```python
from build123d import *

# Parameters (mm, degrees)
F0_R      = 8.37282
F0_R_2    = 8.3693
F1_DEPTH  = 19.05
F2_W      = 20.754474
F2_H      = 61.66184
F3_DEPTH  = 25.4
F5_DEPTH  = 25.4
F7_DEPTH  = 12.7
F6_R      = 3.8309
F8_DEPTH  = 15.24
F10_DEPTH = 12.7
F9_R      = 3.8354
F11_DEPTH = 15.24


with BuildPart() as f1:
    # F0 (on Top) → F1 (new body)
    with BuildSketch(Plane.XY):
        with BuildLine():
            Line((-15.24, 50.8), (-15.24, 0))
            Line((-15.24, 0), (-15.24, -50.8))
            ThreePointArc((-15.24, -50.8), (0, -66.04), (15.24, -50.8))
            Line((15.24, -50.8), (15.24, 0))
            Line((15.24, 0), (15.24, 50.8))
            ThreePointArc((15.24, 50.8), (0, 66.04), (-15.24, 50.8))
        make_face()
        with Locations((0, -50.8)):
            Circle(F0_R, mode=Mode.SUBTRACT)
        with Locations((0, 50.8)):
            Circle(F0_R_2, mode=Mode.SUBTRACT)
    extrude(amount=F1_DEPTH)

    # F2 (on face) → F3 (join)
    with BuildSketch(Plane.XY.offset(19.05)):
        Rectangle(F2_W, F2_H)
    extrude(amount=F3_DEPTH)

    # F4 (on face) → F5 (cut)
    with BuildSketch(Plane.YZ.offset(10.377237)):
        with BuildLine():
            Line((18.13092, 44.45), (-18.13092, 44.45))
            ThreePointArc((-18.13092, 44.45), (0, 27.163165), (18.13092, 44.45))
        make_face()
    extrude(amount=-F5_DEPTH, mode=Mode.SUBTRACT)

    # F6 (on face) → F7 (join)
    with BuildSketch(Plane.XZ.offset(30.83092)):
        with BuildLine():
            Line((3.8309, 44.45), (10.377237, 44.45))
            ThreePointArc((10.377237, 44.45), (0, 54.827237), (-10.377237, 44.45))
            Line((-10.377237, 44.45), (-3.8309, 44.45))
            ThreePointArc((-3.8309, 44.45), (0, 48.2809), (3.8309, 44.45))
        make_face()
    extrude(amount=-F7_DEPTH)

    # F6 (on face) → F8 (cut)
    with BuildSketch(Plane.XZ.offset(30.83092)):
        with Locations((0, 44.45)):
            Circle(F6_R)
    extrude(amount=-F8_DEPTH, mode=Mode.SUBTRACT)

    # F9 (on face) → F10 (join)
    with BuildSketch(Plane(origin=(0, 30.83092, 0), x_dir=(-1, 0, 0), z_dir=(0, 1, 0))):
        with BuildLine():
            Line((3.8354, 44.45), (10.377237, 44.45))
            ThreePointArc((10.377237, 44.45), (0, 54.827237), (-10.377237, 44.45))
            Line((-10.377237, 44.45), (-3.8354, 44.45))
            ThreePointArc((-3.8354, 44.45), (0, 48.2854), (3.8354, 44.45))
        make_face()
    extrude(amount=-F10_DEPTH)

    # F9 (on face) → F11 (cut)
    with BuildSketch(Plane(origin=(0, 30.83092, 0), x_dir=(-1, 0, 0), z_dir=(0, 1, 0))):
        with Locations((0, 44.45)):
            Circle(F9_R)
    extrude(amount=-F11_DEPTH, mode=Mode.SUBTRACT)


solid = f1.part
```
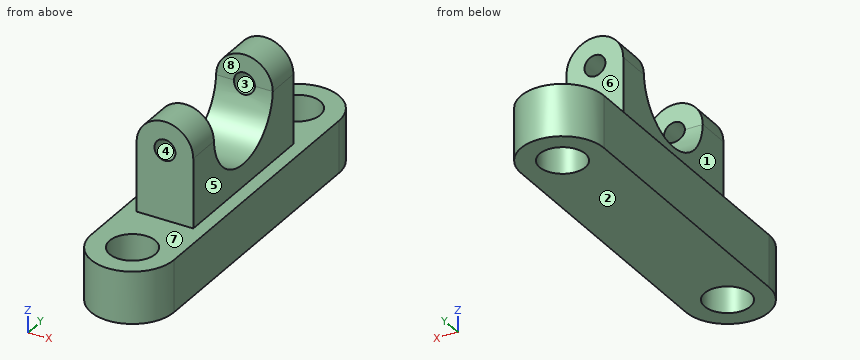
Verification items for the finished model (mm, model axes). Face numbers are marked on the shaded views. A direction names the side the tool comes from. Give positions to 0.01 mm unless a question says otherwise; leave off trailing zeros. Order: outer loops, then holes, each group sorted by start corner. A loop starts at its lowest first (then second) coordinate and runs counter-clockwise, first axis right, second up. Notation, with made-up numbers: (84, -3) -> (102, -3) arc R33 cw to (102, 25) -> close; hole circle Ø10 at (59, -33.5). An arc over 180 degrees is marked (long way). Use a Markdown table: item, result.
1) Section check B-B, the plane z = 5. Record the boundary of the cut face in (x, y).
Results:
| item | result |
|---|---|
| outline | (-15.24, -50.8) arc R15.24 ccw to (15.24, -50.8) -> (15.24, 50.8) arc R15.24 ccw to (-15.24, 50.8) -> close; hole circle Ø16.75 at (0, -50.8); hole circle Ø16.74 at (0, 50.8) |
2) Section check D-D, the plane z = 31.5. Record the boundary of the cut face in (x, y), then the cut area to 3 significant figures.
Results:
| item | result |
|---|---|
| outline | (-10.38, -30.83) -> (10.38, -30.83) -> (10.38, -11.77) -> (-10.38, -11.77) -> close; (-10.38, 11.77) -> (10.38, 11.77) -> (10.38, 30.83) -> (-10.38, 30.83) -> close |
| area | 791 mm² |
3) Mould release check, pull along X, two halves, no side actions. Record for the marked faces 1, 2, 3 and 4: pulls with the +X half, pulls with the -X half, needs draft (parallel to the pull), parting line crosses it, or undercut.
Results:
| item | result |
|---|---|
| face 1 | pulls with the -X half |
| face 2 | needs draft |
| face 3 | undercut |
| face 4 | undercut |
4) Tool access check on the marked faces 5, 6, 7 and 8. Record the directions out of +Z, -Z, +X, -X, +Y, -Y that give a thin tool (end or side, any length) a straight path to the whole face; none if there is none.
Results:
| item | result |
|---|---|
| face 5 | +Z, +X, +Y, -Y |
| face 6 | +Z, +X, -X, +Y |
| face 7 | +Z |
| face 8 | +Z, +X, -X |
5) Depth check by flat-ended pin: pin 1 Ø8.5 at (x, z) = (3.5, 52) entering from +Y; pin 2 Ø4.5 at (x, z) = (0, 44.45) entering from +Y; pin 3 Ø8 at (x, y) = (-4, -38) entering from +Z; pin 4 Ø3 at (x, y) = (-11, -9.5) entering from +Z. Enter the tip coordinate at first touch or a pass-through.
Results:
| item | result |
|---|---|
| pin 1 | y = 30.83 |
| pin 2 | through |
| pin 3 | z = 19.05 |
| pin 4 | z = 30.77 |
6) Section check C-C, the plane y = -47.5. Record the boundary of the cut face in (x, z), then the cut area to 3 significant figures.
Results:
| item | result |
|---|---|
| outline | (-15.24, 0) -> (-7.7, 0) -> (-7.7, 19.05) -> (-15.24, 19.05) -> close; (7.7, 0) -> (15.24, 0) -> (15.24, 19.05) -> (7.7, 19.05) -> close |
| area | 287 mm² |
7) Section check A-A, the plane x = 0. Record the boundary of the cut face in (y, z), then the cut area to 3 significant figures.
Results:
| item | result |
|---|---|
| outline | (-66.04, 0) -> (-59.17, 0) -> (-59.17, 19.05) -> (-66.04, 19.05) -> close; (-42.43, 0) -> (42.43, 0) -> (42.43, 19.05) -> (30.83, 19.05) -> (30.83, 40.61) -> (17.53, 40.61) arc R18.15 cw to (-17.53, 40.62) -> (-30.83, 40.62) -> (-30.83, 19.05) -> (-42.43, 19.05) -> close; (-30.83, 48.28) -> (-18.13, 48.28) -> (-18.13, 54.83) -> (-30.83, 54.83) -> close; (18.13, 48.29) -> (30.83, 48.29) -> (30.83, 54.83) -> (18.13, 54.83) -> close; (59.17, 0) -> (66.04, 0) -> (66.04, 19.05) -> (59.17, 19.05) -> close |
| area | 3,030 mm² |
8) Material ranges on probe 1 along Y at (x, z) = (0, 12); probe 2 along Y at (x, z) = (3.5, 47.5); probe 3 along Z at (x, y) = (0, 27), recorded low to high.
Results:
| item | result |
|---|---|
| probe 1 | -66.04 to -59.17, -42.43 to 42.43, 59.17 to 66.04 |
| probe 2 | -30.83 to -18.13, 18.13 to 30.83 |
| probe 3 | 0 to 40.61, 48.29 to 54.83 |
